Geometry: see drawing. Coordinates: mm, zero at the bounding-box minimum. A direction names the side the tool comes from. Give positions to 0.01 mm unless a question says otherwise; leave off trailing zeros. Write each loop counter-clockwise with the first axis right and the second up, starting at its lowest first coordinate (ties: lowest second). Pieces come first, ordered by that corner, then holes. Notation, with made-up numbers: (87, -21) -> (143, -21) arc R27 ccw to (143, -2) -> close; hole circle Ø10 at (20, -8.75). An arc over 180 degrees is marked (long way). Use CSV: the item, a comma, the result in double quotes. Start each with the question number.
1) Contact query for flat-ended pins moving along their axis: P1, Ø1, axis at y = 6, z = 4, coming from the +X side; P2, Ø4, axis at x = 11, z = 4.5, coming from the -Y side; P3, Ø1.5, axis at x = 24.5, y = 8.5, coming from the +Z side. Output: stop coordinate, or through.
2) Material intervals for line 1 (Y direction, x = 14, z = 1.6); line 2 (Z direction, x = 11.25, y = 3.75); line 3 (Y direction, x = 3, z = 3), sorted ascending. Write a range as [from, to].
3) Section B-B (z = 1.5). Output: boundary loops of the cut face in (x, y), plus the area to 3 significant figures.
4) Section D-D (y = 25). Output: boundary loops of the cut face in (x, z), plus the area to 3 significant figures.
5) Set-up query: the marked faces 4 and 5. Return all of +Z, -Z, +X, -X, +Y, -Y with unobstructed straight access to the full face (end or side cutting, diameter ignored); none if empty.
6) Section C-C (y = 14). Output: boundary loops of the cut face in (x, z).
7) Section A-A (x = 14). Output: boundary loops of the cut face in (y, z).
8) Draft query along Y for the marked faces 1, 2 and 3. Return one class per face: pulls with the +Y half, pulls with the -Y half, needs draft (parallel to the pull), parting line crosses it, or undercut.
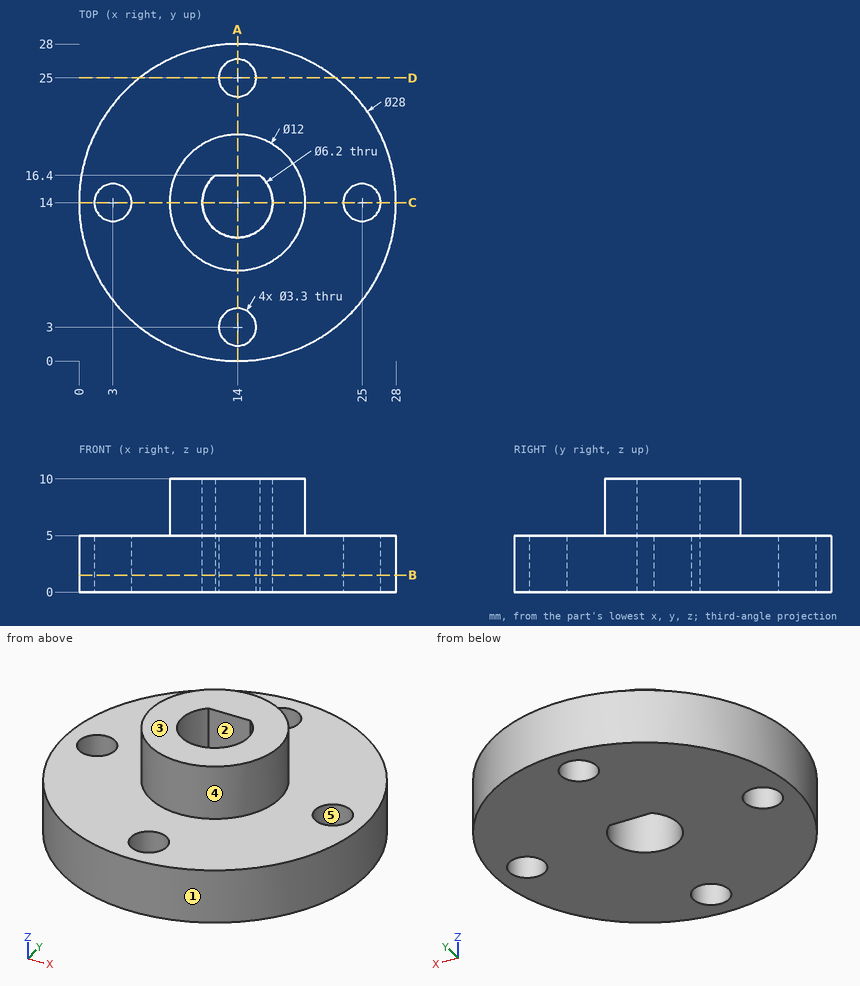
Answers follow:
1,P1,"stops at x = 25.82"
1,P2,"stops at y = 0.04"
1,P3,"stops at z = 5"
2,line 1,"y = [0, 1.35], [4.65, 10.9], [16.4, 23.35], [26.65, 28]"
2,line 2,"z = [0, 5]"
2,line 3,"y = [5.34, 12.35], [15.65, 22.66]"
3,outline,"circle Ø28 at (14, 14); hole circle Ø3.3 at (3, 14); hole (12.04, 16.4) arc R3.1 ccw (long way) to (15.96, 16.4) -> close; hole circle Ø3.3 at (14, 3); hole circle Ø3.3 at (14, 25); hole circle Ø3.3 at (25, 14)"
3,area,"553 mm^2"
4,outline,"(5.34, 0) -> (12.35, 0) -> (12.35, 5) -> (5.34, 5) -> close; (15.65, 0) -> (22.66, 0) -> (22.66, 5) -> (15.65, 5) -> close"
4,area,"70.1 mm^2"
5,face 4,"+Z"
5,face 5,"+Z, -Z"
6,outline,"(0, 0) -> (1.35, 0) -> (1.35, 5) -> (0, 5) -> close; (4.65, 0) -> (10.9, 0) -> (10.9, 10) -> (8, 10) -> (8, 5) -> (4.65, 5) -> close; (17.1, 0) -> (23.35, 0) -> (23.35, 5) -> (20, 5) -> (20, 10) -> (17.1, 10) -> close; (26.65, 0) -> (28, 0) -> (28, 5) -> (26.65, 5) -> close"
7,outline,"(0, 0) -> (1.35, 0) -> (1.35, 5) -> (0, 5) -> close; (4.65, 0) -> (10.9, 0) -> (10.9, 10) -> (8, 10) -> (8, 5) -> (4.65, 5) -> close; (16.4, 0) -> (23.35, 0) -> (23.35, 5) -> (20, 5) -> (20, 10) -> (16.4, 10) -> close; (26.65, 0) -> (28, 0) -> (28, 5) -> (26.65, 5) -> close"
8,face 1,"parting line crosses it"
8,face 2,"undercut"
8,face 3,"needs draft"
